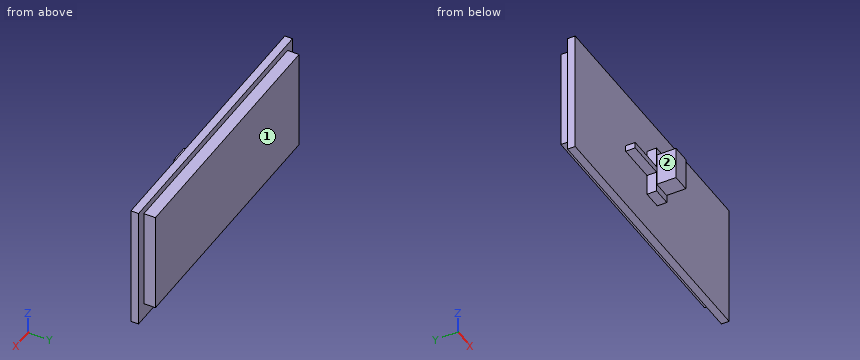
Autodesk Inventor part; units mm, degrees
ref_plane "YZ Plane" through (0, 0, 0) normal (1, 0, 0) x (0, 1, 0)
ref_plane "XZ Plane" through (0, 0, 0) normal (0, 1, 0) x (-1, 0, 0)
ref_plane "XY Plane" through (0, 0, 0) normal (0, 0, 1) x (1, 0, 0)
sketch "Sketch1" plane through (0, 0, 0) normal (0, 1, 0) x (-1, 0, 0)
  line L0 (0, 0) -> (-182.88, 0)
  line L1 (-182.88, 0) -> (-182.88, -82.55)
  line L2 (-182.88, -82.55) -> (0, -82.55)
  line L3 (0, -82.55) -> (0, 0)
  dimension "d0" = 82.55
  dimension "d1" = 182.88
extrude "Extrusion1" add sketch "Sketch1" along normal blind 5.08
sketch "Sketch2" plane through (0, 5.08, 0) normal (0, 1, 0) x (1, 0, 0)
  line L0 (5.842, 71.882) -> (176.53, 71.882)
  line L1 (176.53, 71.882) -> (176.53, 4.572)
  line L2 (176.53, 4.572) -> (5.842, 4.572)
  line L3 (5.842, 4.572) -> (5.842, 71.882)
  line L4 (0, 82.55) -> (0, 0)
  line L5 (182.88, 0) -> (182.88, 82.55)
  line L6 (0, 0) -> (182.88, 0)
  line L7 (182.88, 82.55) -> (0, 82.55)
  line L8 (172.232, 67.584) -> (10.14, 67.584)
  line L9 (10.14, 67.584) -> (10.14, 8.87)
  line L10 (10.14, 8.87) -> (172.232, 8.87)
  line L11 (172.232, 8.87) -> (172.232, 67.584)
  point P0 (182.88, 41.275)
  dimension "d4" = 5.842
  dimension "d5" = 6.35
  dimension "d6" = 4.572
  dimension "d7" = 10.668
extrude "Extrusion2" add sketch "Sketch2" along normal blind 7.62 contours L0 L1 L2 L3 | L11 L10 L9 L8
sketch "Sketch3" plane through (0, 0, 0) normal (0, -1, 0) x (1, 0, 0)
  line L0 (97.536, -57.277) -> (85.344, -57.277)
  line L1 (85.344, -57.277) -> (85.344, -25.273)
  line L2 (85.344, -25.273) -> (97.536, -25.273)
  line L3 (97.536, -25.273) -> (97.536, -57.277)
  line L4 (182.88, 0) -> (182.88, -82.55)
  line L5 (0, 0) -> (182.88, 0)
  line L6 (85.344, -43.307) -> (59.944, -43.307)
  line L7 (59.944, -43.307) -> (59.944, -39.243)
  line L8 (59.944, -39.243) -> (85.344, -39.243)
  line L9 (85.344, -39.243) -> (85.344, -43.307)
  point P0 (97.536, -41.275)
  point P1 (182.88, -41.275)
  point P2 (91.44, -25.273)
  point P3 (91.44, 0)
  point P4 (59.944, -41.275)
  point P5 (85.344, -41.275)
  dimension "d10" = 32.004
  dimension "d11" = 12.192
  dimension "d12" = 25.4
  dimension "d13" = 4.064
extrude "Extrusion3" add sketch "Sketch3" along normal blind 6.35
sketch "Sketch4" plane through (0, -6.35, 0) normal (0, -1, 0) x (1, 0, 0)
  line L0 (97.282, -52.197) -> (85.598, -52.197)
  line L1 (85.598, -52.197) -> (85.598, -30.353)
  line L2 (85.598, -30.353) -> (97.282, -30.353)
  line L3 (97.282, -30.353) -> (97.282, -52.197)
  line L4 (97.536, -57.277) -> (97.536, -25.273)
  line L5 (85.344, -57.277) -> (97.536, -57.277)
  point P0 (0, 0)
  point P1 (85.598, -41.275)
  point P2 (97.536, -41.275)
  point P3 (91.44, -52.197)
  point P4 (91.44, -57.277)
  dimension "d16" = 21.844
  dimension "d17" = 11.684
extrude "Extrusion4" add sketch "Sketch4" along normal blind 12.7
properties part number "Base Box Lid"
Geometry check sheet. Reference: the model listing, model coordinates, mm. Face numbers are marked on the shaded views. A direction names the side the tool comes from. Coordinates: 2 decimals unless noted, no trailing zeros. Order: outer loops, then holes, each group sorted by start corner. A loop starts at its lowest first (then second) coordinate and runs counter-clockwise, first axis right, second up. Notation, with made-up numbers: (29.5, 80) -> (76.5, 80) arc R25 ccw to (76.5, 107) -> close; hole circle Ø2 at (60.25, 25.5). An arc over 180 degrees is marked (long way). Use a Markdown table: item, result. Add a question column.
1. Cross-section at C-C (y = 8). Enter the section's corners in (x, z).
2. Go/stop test with flat-tipped pins: pin 1 Ø8 at (x, y) = (60, -9) entering from -Z; pin 2 Ø7 at (y, z) = (-2.5, -53) entering from -X; pin 3 Ø3.5 at (x, y) = (91, -10.5) entering from -Z; pin 4 Ø1 at (x, y) = (153, 7.5) entering from -Z. Record where each tip stops, or that it passes through.
3. Cross-section at D-D (z = -67.5). Enter the section's corners in (x, y), and give its area (3 significant figures).
4. Material ranges on L1, parallel to X at y = 9.5, z = -50.5; L2, parallel to Y at x = 24, z = -73.5; L3, parallel to Y at x = 28.5, z = -30, recorded low to high.
5. Cross-section at B-B (z = -35). Enter the section's corners in (x, y).
6. Cross-section at A-A (x = 107). Enter the section's corners in (y, z), and give its area (3 significant figures).
7. Set-up check for the marked faces 1 and 2: record each of +Z, -Z, +X, -X, +Y, -Y from which the full face is reachable in a straight line by a thin tool's end or side.
Filled sheet:
| question | item | result |
|---|---|---|
| 1 | outline | (5.84, -71.88) -> (176.53, -71.88) -> (176.53, -4.57) -> (5.84, -4.57) -> close |
| 2 | pin 1 | z = -43.31 |
| 2 | pin 2 | x = 0 |
| 2 | pin 3 | z = -52.2 |
| 2 | pin 4 | z = -71.88 |
| 3 | outline | (0, 0) -> (182.88, 0) -> (182.88, 5.08) -> (176.53, 5.08) -> (176.53, 12.7) -> (5.84, 12.7) -> (5.84, 5.08) -> (0, 5.08) -> close |
| 3 | area | 2,230 mm2 |
| 4 | L1 | 5.84 to 176.53 |
| 4 | L2 | 0 to 5.08 |
| 4 | L3 | 0 to 12.7 |
| 5 | outline | (0, 0) -> (85.34, 0) -> (85.34, -6.35) -> (85.6, -6.35) -> (85.6, -19.05) -> (97.28, -19.05) -> (97.28, -6.35) -> (97.54, -6.35) -> (97.54, 0) -> (182.88, 0) -> (182.88, 5.08) -> (176.53, 5.08) -> (176.53, 12.7) -> (5.84, 12.7) -> (5.84, 5.08) -> (0, 5.08) -> close |
| 6 | outline | (0, -82.55) -> (5.08, -82.55) -> (5.08, -71.88) -> (12.7, -71.88) -> (12.7, -4.57) -> (5.08, -4.57) -> (5.08, 0) -> (0, 0) -> close |
| 6 | area | 932 mm2 |
| 7 | face 1 | +Z, -Z, +X, -X, +Y |
| 7 | face 2 | +Z, -Z, -X, -Y |
